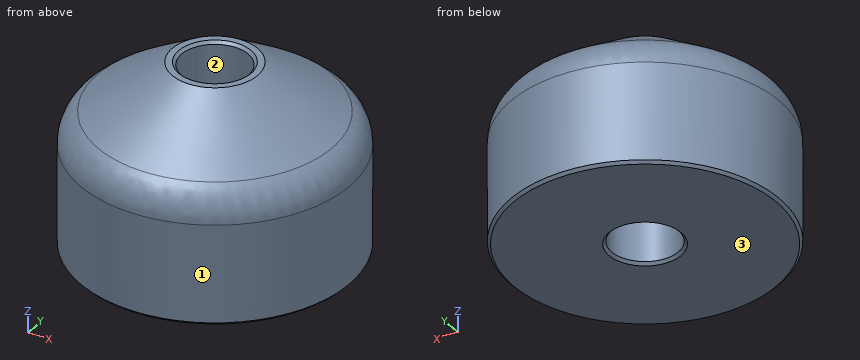
```python
from build123d import *

# Parameters (mm, degrees)
F2_SIZE = 0.175
F3_R    = 2.5


with BuildPart() as f1:
    # F0 (on Right) → F1 (revolve)
    with BuildSketch(Plane.YZ):
        Polygon((-8.65, 7.773333), (-8.65, 0), (-2.15, 0), (-2.15, 11.66), (-2.75, 11.66), align=None)
    revolve(axis=Axis((0, 0, 8.606664), (0, 0, -1)))

    # F2
    f2_edges = [f1.edges().sort_by_distance(p)[0] for p in [
        (0, 2.15, 11.66),
        (0, 8.65, 0),
        (0, 2.15, 0),
    ]]
    chamfer(f2_edges, length=F2_SIZE)

    # F3
    f3_edges = [f1.edges().sort_by_distance(p)[0] for p in [
        (0, 8.65, 7.773333),
    ]]
    fillet(f3_edges, radius=F3_R)


solid = f1.part
```
The model under review builds one solid part; all positions refer to its coordinate system, in mm. Face numbers are marked on the shaded views. Coordinates: 2 decimals unless noted, no trailing zeros. Write each loop counter-clockwise with the first axis right and the second up, starting at its lowest first coordinate (ties: lowest second). Pieces come first, ordered by that corner, then holes. Notation, with made-up numbers: (4, 43.5) -> (43, 43.5) arc R15 cw to (43, 66.5) -> close; hole circle Ø11 at (-7, 11.5). An arc over 180 degrees is marked (long way). One line per item, written item: value. Start each with the question number.
Q1. Clearance check with flat-ended pins moving along their axes: P1, Ø1, axis at y = -2.5, z = 5, coming from the -X side; P2, Ø6, axis at y = -1.5, z = 9.5, coming from the +X side; P3, Ø4, axis at y = -3, z = 10.5, coming from the -X side. State where each tip first meets the part, or that it passes through.
Q2. To check wall thickness, follow probe 1 along Y at (x, z) = (0, 5); probe 2 along X at (y, z) = (0, 8.5). State the ranges of each line that lie inside material, in increasing order.
Q3. Add section A-A, the plane z = 3.25. Give the boundary of the cut face in (x, y), then the cut area to 3 significant figures.
Q4. The part is to be moulded in two halves that separate along X. For the marked faces 1, 2 and 3, say which applies: +X half, -X half, draft (parallel to the pull), parting line (faces both ways), or undercut.
Response:
1. P1: x = -8.42
1. P2: x = 8.62
1. P3: x = -7.02
2. probe 1: -8.65 to -2.15, 2.15 to 8.65
2. probe 2: -7.55 to -2.15, 2.15 to 7.55
3. outline: circle Ø17.3 at (0, 0); hole circle Ø4.3 at (0, 0)
3. area: 221 mm²
4. face 1: parting line
4. face 2: undercut
4. face 3: draft
